The model under review builds one solid part; all positions refer to its coordinate system, in mm. A direction names the side the tool comes from. Round coordinates to 2 decimals unless told otherwise and drop trailing zeros. Order: outer loops, then holes, each group sorted by start corner. A loop starts at its lowest first (then second) coordinate and runs counter-clockwise, first axis right, second up. Notation, with made-up numbers: (88.25, 85) -> (107.25, 85) arc R37 cw to (107.25, 122) -> close; hole circle Ø8 at (8, -5.5). An arc over 180 degrees is marked (long way). Use a Markdown table: item, result. Add a question column.
```python
from build123d import *

# Parameters (mm, degrees)
F1_DEPTH = 90
F3_DEPTH = 2
F4_R     = 3
F6_DEPTH = 3
F7_R     = 1.804785
F7_R_2   = 1.602006
F8_DEPTH = 3


with BuildPart() as f1:
    # F0 (on Front) → F1 (new body)
    with BuildSketch(Plane.XZ):
        with BuildLine():
            Line((24, 0), (26, 0))
            ThreePointArc((26, 0), (0, 26), (-26, 0))
            Line((-26, 0), (-24, 0))
            ThreePointArc((-24, 0), (0, 24), (24, 0))
        make_face()
    extrude(amount=F1_DEPTH)

    # F2 (on face) → F3 (join)
    with BuildSketch(Plane.XZ.offset(90)):
        with BuildLine():
            Line((-26, 0), (26, 0))
            ThreePointArc((26, 0), (0, 26), (-26, 0))
        make_face()
    extrude(amount=F3_DEPTH)

    # F4
    f4_edges = [f1.edges().sort_by_distance(p)[0] for p in [
        (0, -92, 26),
    ]]
    fillet(f4_edges, radius=F4_R)

    # F5 (on Front) → F6 (join)
    with BuildSketch(Plane.XZ):
        with BuildLine():
            Line((-26, 0), (26, 0))
            ThreePointArc((26, 0), (0, 26), (-26, 0))
        make_face()
    extrude(amount=F6_DEPTH)

    # F7 (on face) → F8 (cut)
    with BuildSketch(Plane(origin=(0, 0, 0), x_dir=(-1, 0, 0), z_dir=(0, 1, 0))):
        with Locations((0, 16.952889)):
            Circle(F7_R)
        with Locations((15.691938, 6.337816)):
            Circle(F7_R_2)
        with Locations((-15.691938, 6.337816)):
            Circle(F7_R_2)
    extrude(amount=-F8_DEPTH, mode=Mode.SUBTRACT)


solid = f1.part
```
Q1. For pin 1 (1.5 mm diameter, centred on x = -3, y = -20.5, fed in from -Z); pin 2 (3 mm diameter, centred on x = 4.5, y = -66, fed in from -Z); pin 3 (4 mm diameter, centred on x = -19.5, y = -49, fed in from +Z), all flat-tipped, find the tip position at first contact; note any pin that passes through.
Q2. To check wall thickness, follow line 1 along Y through (x, z) = (-7.5, 6.5); line 2 along X through (y, z) = (-61, 21.5); line 3 along Z through (x, y) = (0.5, -17). State the ranges of each line that lie inside material, in increasing order.
Q3. Draft analysis for pull direction Y (two halves, no side actions). For faces 4 (the face through (17.292, -1.479, 6.408)), 5 (the face through (0, 0, 10)), 6 (the face through (0, -92, 9)), 7 (the face through (0, -3, 10)), state which applies: released by +Y, released by -Y, zero draft, split by the parting line, or undercut.
Q4. Add section B-B, the plane y = -9. Give the boundary of the cut face in (x, z).
Q5. For faces 1 (the face through (0.572, -43.877, 25.994)), 2 (the face through (0, -90, 10)), 3 (the face through (0.39, -1.48, 15.19)), list the 3-axis set-ups (+Z, -Z, +X, -X, +Y, -Y) from which the entire face can be reached by the end or side of a thin tool; tool diameter is ignored.
Q6. Add section A-A, the plane x = 0. Give the boundary of the cut face in (y, z), then the cut area to 3 significant figures.
Return value:
| question | item | result |
|---|---|---|
| 1 | pin 1 | z = 23.71 |
| 1 | pin 2 | z = 23.24 |
| 1 | pin 3 | z = 19.23 |
| 2 | line 1 | -92 to -90, -3 to 0 |
| 2 | line 2 | -14.62 to -10.67, 10.67 to 14.62 |
| 2 | line 3 | 23.99 to 26 |
| 3 | face 4 | zero draft |
| 3 | face 5 | released by +Y |
| 3 | face 6 | released by -Y |
| 3 | face 7 | undercut |
| 4 | outline | (-26, 0) -> (-24, 0) arc R24 cw to (24, 0) -> (26, 0) arc R26 ccw to start |
| 5 | face 1 | +Z, +Y, -Y |
| 5 | face 2 | -Z |
| 5 | face 3 | +Y |
| 6 | outline | (-92, 0) -> (-90, 0) -> (-90, 24) -> (-3, 24) -> (-3, 18.76) -> (0, 18.76) -> (0, 26) -> (-89, 26) arc R3 ccw to (-92, 23) -> close; (-3, 0) -> (0, 0) -> (0, 15.15) -> (-3, 15.15) -> close |
| 6 | area | 291 mm² |
